from build123d import *

# Parameters (mm, degrees)
BOSS_EXTRUDE1_DEPTH = 20
SKETCH2_W           = 10
SKETCH2_H           = 2
BOSS_EXTRUDE2_DEPTH = 20
SKETCH3_W           = 2.5
SKETCH3_H           = 10
CUT_EXTRUDE1_DEPTH  = 64.695758612
BOSS_EXTRUDE3_START = 5
BOSS_EXTRUDE3_DEPTH = 10
SKETCH15_W          = 9.957494595
SKETCH15_H          = 3.486023066
SKETCH15_W_2        = 10
SKETCH15_H_2        = 3.406795269
CUT_EXTRUDE2_DEPTH  = 4
SKETCH16_R          = 0.429985908
CUT_EXTRUDE3_DEPTH  = 70.31700842
SKETCH19_R          = 0.43
CUT_EXTRUDE4_DEPTH  = 70.31700842


# Read off the part's stored shape, not the designer's step: Boss-Extrude3
with BuildPart() as part:
    # Sketch1 → Boss-Extrude1 (new body)
    with BuildSketch(Plane.XY):
        with BuildLine():
            Line((-44.6875, 2.119473798), (-39.6875, 2.119473798))
            ThreePointArc((-39.6875, 2.119473798), (-9.6875, 32.119473798), (20.3125, 2.119473798))
            Line((20.3125, 2.119473798), (25.232533649, 2.119473798))
            ThreePointArc((25.232533649, 2.119473798), (-9.727483176, 36.591230483), (-44.6875, 2.119473798))
        make_face()
    extrude(amount=BOSS_EXTRUDE1_DEPTH)

    # Sketch2 → Boss-Extrude2 (add)
    with BuildSketch(Plane.XY.offset(20)):
        with Locations((25.3125, 1.119473798)):
            Rectangle(SKETCH2_W, SKETCH2_H)
        with Locations((-44.6875, 1.119473798)):
            Rectangle(SKETCH2_W, SKETCH2_H)
    extrude(amount=-BOSS_EXTRUDE2_DEPTH)

    # Sketch3 → Cut-Extrude1 (cut, through all)
    with BuildSketch(Plane(origin=(0, 2.119473798, 0), x_dir=(1, 0, 0), z_dir=(0, 1, 0))):
        with Locations((-47.1875, -10)):
            Rectangle(SKETCH3_W, SKETCH3_H)
        with Locations((27.628360341, -10)):
            Rectangle(SKETCH3_W, SKETCH3_H)
    extrude(amount=-CUT_EXTRUDE1_DEPTH, mode=Mode.SUBTRACT)

    # Boss-Extrude3 outline → Boss-Extrude3 (add)
    with BuildSketch(Plane.XY.offset(BOSS_EXTRUDE3_START)):
        with BuildLine():
            ThreePointArc((-34.6875, 26.11126295), (-30.002295927, 30.112427643), (-24.6875, 33.229060498))
            Line((-24.6875, 33.229060498), (-24.6875, 44))
            Line((-24.6875, 44), (-34.6875, 44))
            Line((-34.6875, 44), (-34.6875, 26.11126295))
        make_face()
        with BuildLine():
            Line((5.232533649, 44), (5.232533649, 33.229060498))
            ThreePointArc((5.232533649, 33.229060498), (10.547329576, 30.112427643), (15.232533649, 26.11126295))
            Line((15.232533649, 26.11126295), (15.232533649, 44))
            Line((15.232533649, 44), (5.232533649, 44))
        make_face()
    extrude(amount=BOSS_EXTRUDE3_DEPTH)

    # Sketch15 → Cut-Extrude2 (cut)
    with BuildSketch(Plane(origin=(0, 0, 5), x_dir=(-1, 0, 0), z_dir=(0, 0, -1))):
        with Locations((-10.211280947, 38.350092999)):
            Rectangle(SKETCH15_W, SKETCH15_H)
        with Locations((29.6875, 38.389706898)):
            Rectangle(SKETCH15_W_2, SKETCH15_H_2)
    extrude(amount=-CUT_EXTRUDE2_DEPTH, mode=Mode.SUBTRACT)

    # Sketch16 → Cut-Extrude3 (cut, through all)
    with BuildSketch(Plane.XY):
        with Locations((-40.194076416, 2.70790241)):
            Circle(SKETCH16_R)
    extrude(amount=CUT_EXTRUDE3_DEPTH, mode=Mode.SUBTRACT)

    # Sketch19 → Cut-Extrude4 (cut, through all)
    with BuildSketch(Plane(origin=(0, 0, 0), x_dir=(-1, 0, 0), z_dir=(0, 0, -1))):
        with Locations((40.157773316, 3.842579994)):
            Circle(SKETCH19_R)
        with Locations((40.129976485, 4.951475276)):
            Circle(SKETCH19_R)
        with Locations((39.976743657, 6.041690441)):
            Circle(SKETCH19_R)
        with Locations((39.77957363, 7.060618267)):
            Circle(SKETCH19_R)
        with Locations((39.611616001, 8.083648579)):
            Circle(SKETCH19_R)
        with Locations((39.384056604, 9.117159584)):
            Circle(SKETCH19_R)
        with Locations((38.829794547, 11.043164756)):
            Circle(SKETCH19_R)
        with Locations((38.552022228, 12.048984433)):
            Circle(SKETCH19_R)
        with Locations((39.088806217, 10.095021994)):
            Circle(SKETCH19_R)
        with Locations((38.141177141, 12.983497136)):
            Circle(SKETCH19_R)
        with Locations((37.768769018, 13.895051344)):
            Circle(SKETCH19_R)
        with Locations((37.448916338, 14.800008888)):
            Circle(SKETCH19_R)
        with Locations((37.032221222, 15.670387014)):
            Circle(SKETCH19_R)
        with Locations((36.528360395, 16.609796608)):
            Circle(SKETCH19_R)
        with Locations((35.986242339, 17.577737268)):
            Circle(SKETCH19_R)
        with Locations((35.393593155, 18.525538356)):
            Circle(SKETCH19_R)
        with Locations((34.843911912, 19.412863745)):
            Circle(SKETCH19_R)
        with Locations((34.19539752, 20.296560878)):
            Circle(SKETCH19_R)
        with Locations((33.671579827, 21.16369959)):
            Circle(SKETCH19_R)
        with Locations((30.049939441, 24.82228941)):
            Circle(SKETCH19_R)
        with Locations((29.247761657, 25.528887704)):
            Circle(SKETCH19_R)
        with Locations((28.468285707, 26.171032429)):
            Circle(SKETCH19_R)
        with Locations((27.575265581, 26.752789683)):
            Circle(SKETCH19_R)
        with Locations((26.807973066, 27.321370243)):
            Circle(SKETCH19_R)
        with Locations((26.018155923, 27.899111723)):
            Circle(SKETCH19_R)
        with Locations((25.117140803, 28.388278306)):
            Circle(SKETCH19_R)
        with Locations((24.152740884, 28.916859444)):
            Circle(SKETCH19_R)
        with Locations((23.213415748, 29.452693957)):
            Circle(SKETCH19_R)
        with Locations((22.265953613, 29.915077196)):
            Circle(SKETCH19_R)
        with Locations((21.292090137, 30.317791635)):
            Circle(SKETCH19_R)
        with Locations((20.341195492, 30.670660652)):
            Circle(SKETCH19_R)
        with Locations((19.294443445, 31.027159999)):
            Circle(SKETCH19_R)
        with Locations((18.273341346, 31.346527811)):
            Circle(SKETCH19_R)
        with Locations((17.330694676, 31.659064493)):
            Circle(SKETCH19_R)
        with Locations((16.213760043, 31.925126509)):
            Circle(SKETCH19_R)
        with Locations((15.196392743, 32.163250345)):
            Circle(SKETCH19_R)
        with Locations((14.118871826, 32.276097443)):
            Circle(SKETCH19_R)
        with Locations((9.989341485, 32.586591657)):
            Circle(SKETCH19_R)
        with Locations((32.972067882, 21.91183374)):
            Circle(SKETCH19_R)
        with Locations((32.214660672, 22.653461633)):
            Circle(SKETCH19_R)
        with Locations((31.504591412, 23.442427477)):
            Circle(SKETCH19_R)
        with Locations((30.768790829, 24.13924253)):
            Circle(SKETCH19_R)
        with Locations((13.058680454, 32.446158075)):
            Circle(SKETCH19_R)
        with Locations((12.053860203, 32.501632039)):
            Circle(SKETCH19_R)
        with Locations((11.034344787, 32.535615887)):
            Circle(SKETCH19_R)
        with Locations((8.961330107, 32.55260781)):
            Circle(SKETCH19_R)
        with Locations((7.941814691, 32.518623963)):
            Circle(SKETCH19_R)
        with Locations((6.837339657, 32.518623963)):
            Circle(SKETCH19_R)
        with Locations((5.780100612, 32.378387633)):
            Circle(SKETCH19_R)
        with Locations((4.731513778, 32.180229491)):
            Circle(SKETCH19_R)
        with Locations((3.748979658, 32.015097706)):
            Circle(SKETCH19_R)
        with Locations((2.758188948, 31.825196153)):
            Circle(SKETCH19_R)
        with Locations((1.825194364, 31.544472119)):
            Circle(SKETCH19_R)
        with Locations((0.859173422, 31.338057388)):
            Circle(SKETCH19_R)
        with Locations((-0.115104109, 31.016050407)):
            Circle(SKETCH19_R)
        with Locations((-1.097638229, 30.636247302)):
            Circle(SKETCH19_R)
        with Locations((-2.076149977, 30.222346847)):
            Circle(SKETCH19_R)
        with Locations((-3.049992433, 29.818110356)):
            Circle(SKETCH19_R)
        with Locations((-3.950337346, 29.386312285)):
            Circle(SKETCH19_R)
        with Locations((-4.813933487, 28.890203864)):
            Circle(SKETCH19_R)
        with Locations((-5.677529628, 28.412469829)):
            Circle(SKETCH19_R)
        with Locations((-6.550312962, 27.962297372)):
            Circle(SKETCH19_R)
        with Locations((-7.413502609, 27.366093596)):
            Circle(SKETCH19_R)
        with Locations((-8.219973711, 26.777503937)):
            Circle(SKETCH19_R)
        with Locations((-8.986938394, 26.196288512)):
            Circle(SKETCH19_R)
        with Locations((-9.831797929, 25.597097353)):
            Circle(SKETCH19_R)
        with Locations((-10.553062854, 24.903287734)):
            Circle(SKETCH19_R)
        with Locations((-11.310165464, 24.258114165)):
            Circle(SKETCH19_R)
        with Locations((-12.06420723, 23.557388483)):
            Circle(SKETCH19_R)
        with Locations((-12.726849995, 22.772880383)):
            Circle(SKETCH19_R)
        with Locations((-13.381876175, 22.041688367)):
            Circle(SKETCH19_R)
        with Locations((-14.045284633, 21.325390255)):
            Circle(SKETCH19_R)
        with Locations((-14.610568668, 20.575076455)):
            Circle(SKETCH19_R)
        with Locations((-15.160955996, 19.793949768)):
            Circle(SKETCH19_R)
        with Locations((-15.722428913, 18.979418635)):
            Circle(SKETCH19_R)
        with Locations((-16.323442177, 18.141163294)):
            Circle(SKETCH19_R)
        with Locations((-16.861190886, 17.247551468)):
            Circle(SKETCH19_R)
        with Locations((-17.370099884, 16.349117506)):
            Circle(SKETCH19_R)
        with Locations((-17.822461681, 15.472834796)):
            Circle(SKETCH19_R)
        with Locations((-18.259251056, 14.590047971)):
            Circle(SKETCH19_R)
        with Locations((-18.641379366, 13.645130385)):
            Circle(SKETCH19_R)
        with Locations((-19.030723208, 12.71256922)):
            Circle(SKETCH19_R)
        with Locations((-19.316434923, 11.726402977)):
            Circle(SKETCH19_R)
        with Locations((-19.611363146, 10.684937692)):
            Circle(SKETCH19_R)
        with Locations((-19.926919345, 9.635249333)):
            Circle(SKETCH19_R)
        with Locations((-20.1750725, 8.564272558)):
            Circle(SKETCH19_R)
        with Locations((-20.384043578, 7.545538552)):
            Circle(SKETCH19_R)
        with Locations((-20.593014656, 6.526804546)):
            Circle(SKETCH19_R)
        with Locations((-20.697500195, 5.573374003)):
            Circle(SKETCH19_R)
        with Locations((-20.736682272, 4.580761382)):
            Circle(SKETCH19_R)
        with Locations((-20.767815184, 3.558359305)):
            Circle(SKETCH19_R)
        with Locations((-20.808866838, 2.521805048)):
            Circle(SKETCH19_R)
    extrude(amount=-CUT_EXTRUDE4_DEPTH, mode=Mode.SUBTRACT)


solid = part.part
Source: CAD feature listing. Evaluate the final solid. Frame: model axes, mm. A direction names the side the tool comes from. Coordinates: 2 decimals unless noted, no trailing zeros. Write each question's results on one line, items separated by ' | '. Start each with the question number.
Item 1: First-contact query: pin 1 Ø1 at (x, z) = (-20, 13.5) entering from -Y; pin 2 Ø4 at (y, z) = (38, 15.5) entering from -X; pin 3 Ø1 at (y, z) = (15, 14.5) entering from -X; pin 4 Ø6 at (x, y) = (-4, 38.5) entering from +Z. Flat tips, straight axial feed; report the tip coordinate or a pass-through.
Item 2: Line query: probe 1 along Y at (x, z) = (-35.5, 3); probe 2 along X at (y, z) = (42, 11.75); probe 3 along X at (y, z) = (16, 17.25). Output: solid intervals per line, ascending.
Item 3: Set-up query: faces 5 (the face through (10, 35, 5)), 6 (the face through (-39.688, 1, 10)), 7 (the face through (28, 1, 15)), 8 (the face through (10, 37, 15)), 9 (the face through (29.4, 2.119, 10.1)). Return all of +Z, -Z, +X, -X, +Y, -Y with unobstructed straight access to the full face (end or side cutting, diameter ignored); none if empty.
Item 4: Cut plane A-A (z = 6.75). Count the separate pieces of the cut face and the enclosed holes in it, and give its area (3 significant figures).
Item 5: Draft query along X for faces 1 (the face through (15.233, 35, 10)), 2 (the face through (-49, 2.119, 10)), 3 (the face through (-48.438, 1, 10)), 4 (the face through (5.233, 39, 10)). Return one class per face: pulls with the +X half, pulls with the -X half, needs draft (parallel to the pull), parting line crosses it, or undercut.
Checked values:
1) pin 1: stops at y = 30.1 | pin 2: stops at x = -34.69 | pin 3: stops at x = -42.24 | pin 4: stops at z = 20
2) probe 1: y = 17.41 to 18.11, 18.94 to 25.25 | probe 2: x = -34.69 to -24.69, 5.23 to 15.23 | probe 3: x = -41.6 to -37.31, -36.76 to -36.28, 16.91 to 17.12, 17.62 to 22.15
3) face 5: -Z, +X, +Y | face 6: +Z, -Z, -Y | face 7: +Y, -Y | face 8: +Z, +X, +Y | face 9: +Z, -Z, +X, +Y
4) separate pieces: 4 | enclosed holes: 93 | area: 657 mm2
5) face 1: pulls with the +X half | face 2: needs draft | face 3: undercut | face 4: undercut
